from build123d import *

# Parameters (mm, degrees)
SKETCH1_W                 = 43
SKETCH1_H                 = 60
BOSS_EXTRUDE1_DEPTH       = 55
SKETCH2_W                 = 41.9
SKETCH2_H                 = 20
CUT_EXTRUDE1_DEPTH        = 38
SKETCH3_W                 = 9.05
SKETCH3_H                 = 8
CUT_EXTRUDE2_DEPTH        = 38
SKETCH4_W                 = 60
SKETCH4_H                 = 55
CUT_EXTRUDE3_DEPTH        = 13
BOSS_EXTRUDE5_START       = -0.874015748
BOSS_EXTRUDE5_OUTLINE_W   = 2
BOSS_EXTRUDE5_OUTLINE_H   = 41.9
BOSS_EXTRUDE5_OUTLINE_W_2 = 5
BOSS_EXTRUDE5_OUTLINE_H_2 = 20
BOSS_EXTRUDE5_DEPTH       = 30
SKETCH12_R                = 2.55
CUT_EXTRUDE4_DEPTH        = 10
SKETCH13_R                = 2.55
CUT_EXTRUDE5_DEPTH        = 10
SKETCH15_W                = 41.9
SKETCH15_H                = 5
CUT_EXTRUDE7_DEPTH        = 25
SKETCH16_W                = 41.9
SKETCH16_H                = 3
BOSS_EXTRUDE6_DEPTH       = 25


# Read off the part's stored shape, not the designer's step: Boss-Extrude5
with BuildPart() as part:
    # Sketch1 → Boss-Extrude1 (new body)
    with BuildSketch(Plane(origin=(0, 0, 0), x_dir=(1, 0, 0), z_dir=(0, 1, 0))):
        with Locations((20.625984252, 7.362204724)):
            Rectangle(SKETCH1_W, SKETCH1_H)
    extrude(amount=BOSS_EXTRUDE1_DEPTH)

    # Sketch2 → Cut-Extrude1 (cut)
    with BuildSketch(Plane(origin=(42.125984252, 0, 0), x_dir=(0, 0, -1), z_dir=(1, 0, 0))):
        with Locations((7.362204724, 40.5)):
            Rectangle(SKETCH2_W, SKETCH2_H)
        with Locations((7.362204724, 15)):
            Rectangle(SKETCH2_W, SKETCH2_H)
    extrude(amount=-CUT_EXTRUDE1_DEPTH, mode=Mode.SUBTRACT)

    # Sketch3 → Cut-Extrude2 (cut)
    with BuildSketch(Plane(origin=(42.125984252, 0, 0), x_dir=(0, 0, -1), z_dir=(1, 0, 0))):
        with Locations((-18.112795276, 15)):
            Rectangle(SKETCH3_W, SKETCH3_H)
        with Locations((32.837204724, 40.5)):
            Rectangle(SKETCH3_W, SKETCH3_H)
    extrude(amount=-CUT_EXTRUDE2_DEPTH, mode=Mode.SUBTRACT)

    # Sketch4 → Cut-Extrude3 (cut)
    with BuildSketch(Plane(origin=(42.125984252, 0, 0), x_dir=(0, 0, -1), z_dir=(1, 0, 0))):
        with Locations((7.362204724, 27.5)):
            Rectangle(SKETCH4_W, SKETCH4_H)
    extrude(amount=-CUT_EXTRUDE3_DEPTH, mode=Mode.SUBTRACT)

    # Boss-Extrude5 outline → Boss-Extrude5 (add)
    with BuildSketch(Plane.YZ.offset(BOSS_EXTRUDE5_START)):
        with Locations((6, -7.362204724)):
            Rectangle(BOSS_EXTRUDE5_OUTLINE_W, BOSS_EXTRUDE5_OUTLINE_H)
        with Locations((4.5, -47.362204724)):
            Rectangle(BOSS_EXTRUDE5_OUTLINE_W_2, BOSS_EXTRUDE5_OUTLINE_H_2)
        with Locations((4.5, 32.637795276)):
            Rectangle(BOSS_EXTRUDE5_OUTLINE_W_2, BOSS_EXTRUDE5_OUTLINE_H_2)
    extrude(amount=BOSS_EXTRUDE5_DEPTH)

    # Sketch12 → Cut-Extrude4 (cut)
    with BuildSketch(Plane(origin=(29.125984252, 0, 0), x_dir=(0, 0, -1), z_dir=(1, 0, 0))):
        with Locations((-17.437795276, 45.5)):
            Circle(SKETCH12_R)
        with Locations((-17.437795276, 35.5)):
            Circle(SKETCH12_R)
    extrude(amount=-CUT_EXTRUDE4_DEPTH, mode=Mode.SUBTRACT)

    # Sketch13 → Cut-Extrude5 (cut)
    with BuildSketch(Plane(origin=(29.125984252, 0, 0), x_dir=(0, 0, -1), z_dir=(1, 0, 0))):
        with Locations((32.162204724, 20)):
            Circle(SKETCH13_R)
        with Locations((32.162204724, 10)):
            Circle(SKETCH13_R)
    extrude(amount=-CUT_EXTRUDE5_DEPTH, mode=Mode.SUBTRACT)

    # Sketch15 → Cut-Extrude7 (cut)
    with BuildSketch(Plane(origin=(29.125984252, 0, 0), x_dir=(0, 0, -1), z_dir=(1, 0, 0))):
        with Locations((7.362204724, 4.5)):
            Rectangle(SKETCH15_W, SKETCH15_H)
    extrude(amount=-CUT_EXTRUDE7_DEPTH, mode=Mode.SUBTRACT)

    # Sketch16 → Boss-Extrude6 (add)
    with BuildSketch(Plane(origin=(4.125984252, 0, 0), x_dir=(0, 0, -1), z_dir=(1, 0, 0))):
        with Locations((7.362204724, 3.5)):
            Rectangle(SKETCH16_W, SKETCH16_H)
    extrude(amount=BOSS_EXTRUDE6_DEPTH)


solid = part.part
Design review of the part built by this model. Coordinates are the model's own, in mm. A direction names the side the tool comes from. Give positions to 0.01 mm unless a question says otherwise; leave off trailing zeros. Loops run counter-clockwise (first coordinate to the right, second up) from the corner with the lowest first, then second, coordinate; pieces in that order, holes last. Notation, with made-up numbers: M 12,41 L 43,41 A32 ccw 43,80 Z; hole C -34.5,26.5 d7. An arc over 180 degrees is marked long. Write item = value, one per line.
Q1. To check wall thickness, follow line 1 (Y direction, x = 9, z = -24.5); line 2 (Z direction, x = 24, y = 35); line 3 (Z direction, x = 5, y = 8.5). State the ranges of each line that lie inside material, in increasing order. Write a range as [from, to].
Output values:
line_1 = [0, 5], [25, 30.5], [50.5, 55]
line_2 = [-37.36, -28.31], [13.59, 14.94], [19.94, 22.64]
line_3 = [-37.36, -28.31], [13.59, 22.64]
Q2. We need section B-B (x = 26.5). Count the separate pieces of the cut face and the enclosed holes in it, plus the area to 3 significant figures.
Output values:
separate_pieces = 1
enclosed_holes = 4
area = 1,600 mm^2
Q3. Insertion check: pin 1 (4 mm diameter, centred on x = 24.5, z = 25, fed in from -Y); pin 2 (0.6 mm diameter, centred on x = 20.5, y = 1.5, fed in from -Z); pin 3 (6 mm diameter, centred on y = 19.5, z = 3, fed in from +X). Each pin has a flat end and moves straight along its axis. Give the tip position at first contact, or say it passes through.
Output values:
pin_1 = 2
pin_2 = -37.36
pin_3 = 4.13
Q4. We need section D-D (z = -39.5). Give the boundary of the cut face in (x, y).
Output values:
outline = M -0.87,2 L 29.13,2 L 29.13,7 L -0.87,7 Z
Q5. We need section A-A (y = 10). Give the boundary of the cut face in (x, z).
Output values:
outline = M -0.87,-37.36 L 29.13,-37.36 L 29.13,-34.71 L 19.13,-34.71 L 19.13,-29.61 L 29.13,-29.61 L 29.13,-28.31 L 4.13,-28.31 L 4.13,13.59 L 29.13,13.59 L 29.13,22.64 L -0.87,22.64 Z
Q6. Draft analysis for pull direction Z (two halves, no side actions). For faces 1 (the cylindrical face through (24.2, 38.03, 17.77)), 2 (the flat face through (14, 31, 22.638)), 3 (the flat face through (14, 7, -48)), state which applies: +Z half, -Z half, draft (parallel to the pull), parting line (faces both ways), or undercut.
Output values:
face_1 = undercut
face_2 = +Z half
face_3 = draft
Q7. For faces 4 (the flat face through (17, 11, 18)), 5 (the flat face through (14, 2, 32)), 6 (the flat face through (14, 31, -37.362)), 7 (the flat face through (16, 5, -7)), list the 3-axis set-ups (+Z, -Z, +X, -X, +Y, -Y) from which the entire face can be reached by the end or side of a thin tool; tool diameter is ignored.
Output values:
face_4 = +Z, +X
face_5 = +Z, +X, -X, -Y
face_6 = -Z, +X, -X, +Y
face_7 = +X
Q8. We need section C-C (x = 18). Give the boundary of the cut face in (y, z), plus the area to 3 significant figures.
Output values:
outline = M 0,-37.36 L 2,-37.36 L 2,-57.36 L 7,-57.36 L 7,-37.36 L 36.5,-37.36 L 36.5,-28.31 L 30.5,-28.31 L 30.5,13.59 L 50.5,13.59 L 50.5,-28.31 L 44.5,-28.31 L 44.5,-37.36 L 55,-37.36 L 55,22.64 L 19,22.64 L 19,13.59 L 25,13.59 L 25,-28.31 L 5,-28.31 L 5,13.59 L 11,13.59 L 11,22.64 L 7,22.64 L 7,42.64 L 2,42.64 L 2,22.64 L 0,22.64 Z
area = 1,680 mm^2
